from build123d import *

# Parameters (mm, degrees)
BOSS_EXTRUDE1_DEPTH = 0.75
BOSS_EXTRUDE2_DEPTH = 0.5
CUT_EXTRUDE1_DEPTH  = 0.1
CUT_EXTRUDE2_DEPTH  = 0.2
SKETCH5_W           = 0.45
SKETCH5_H           = 0.6
SKETCH6_W           = 0.45
SKETCH6_H           = 0.6
SKETCH7_W           = 1.25
SKETCH7_H           = 0.5
HOLE1_D             = 0.9
HOLE1_DEPTH         = 1.85
HOLE1_CBORE_D       = 2.5
HOLE1_CBORE_DEPTH   = 0.75
FILLET1_R           = 0.1
CHAMFER1_SIZE       = 0.15
FILLET2_R           = 0.25
FILLET3_R           = 1


with BuildPart() as part:
    # Sketch1 → Boss-Extrude1 (new body)
    with BuildSketch(Plane(origin=(0, 0, 0), x_dir=(-1, 0, 0), z_dir=(0, 0, -1))):
        with BuildLine():
            Line((-18.147160188, -0.321056231), (-16.640459832, -0.807555039))
            ThreePointArc((-16.640459832, -0.807555039), (-14.376672703, 1.830313994), (-11.123104682, 3.053988922))
            Line((-11.123104682, 3.053988922), (-11.854774008, 4.687962623))
            Line((-11.854774008, 4.687962623), (-11.980143643, 8.966094329))
            Line((-11.980143643, 8.966094329), (-13.651153285, 11.372867219))
            ThreePointArc((-13.651153285, 11.372867219), (-13.886856414, 11.501581597), (-14.131154362, 11.390038472))
            ThreePointArc((-14.131154362, 11.390038472), (-17.168571063, 5.887500969), (-18.147160188, -0.321056231))
        make_face()
    extrude(amount=-BOSS_EXTRUDE1_DEPTH)

    # Sketch2 → Boss-Extrude2 (add)
    with BuildSketch(Plane.XY.offset(0.75)):
        with BuildLine():
            Line((18.147160188, -0.321056231), (16.196912485, -0.950772139))
            Line((16.196912485, -0.950772139), (13.090029226, -4.428012343))
            Line((13.090029226, -4.428012343), (12.448174494, -4.428012343))
            ThreePointArc((12.448174494, -4.428012343), (9.659124877, -5.936170482), (8.400603878, -3.02593619))
            Line((8.400603878, -3.02593619), (11.854774008, 4.687962623))
            Line((11.854774008, 4.687962623), (11.980143643, 8.966094329))
            Line((11.980143643, 8.966094329), (13.651153285, 11.372867219))
            ThreePointArc((13.651153285, 11.372867219), (13.886856414, 11.501581597), (14.131154362, 11.390038472))
            ThreePointArc((14.131154362, 11.390038472), (17.168571063, 5.887500969), (18.147160188, -0.321056231))
        make_face()
    extrude(amount=BOSS_EXTRUDE2_DEPTH)

    # Sketch3 → Cut-Extrude1 (cut)
    with BuildSketch(Plane.XY.offset(1.25)):
        with BuildLine():
            Line((11.118831997, 2.571420588), (10.212805559, -1.893755119))
            Line((10.212805559, -1.893755119), (9.327068413, -3.204862093))
            ThreePointArc((9.327068413, -3.204862093), (11.06260071, -2.868815002), (11.3986478, -4.604347299))
            Line((11.3986478, -4.604347299), (12.284384946, -3.293240325))
            Line((12.284384946, -3.293240325), (16.088661421, -0.786019055))
            ThreePointArc((16.088661421, -0.786019055), (14.012715525, 1.498074346), (11.118831997, 2.571420588))
        make_face()
    extrude(amount=-CUT_EXTRUDE1_DEPTH, mode=Mode.SUBTRACT)

    # Sketch4 → Cut-Extrude2 (cut)
    with BuildSketch(Plane.XY.offset(1.15)):
        with BuildLine():
            Line((11.006450661, -0.718966828), (9.327068413, -3.204862093))
            ThreePointArc((9.327068413, -3.204862093), (11.06260071, -2.868815002), (11.3986478, -4.604347299))
            Line((11.3986478, -4.604347299), (13.078030048, -2.118452035))
            ThreePointArc((13.078030048, -2.118452035), (12.182188875, -1.211551493), (11.006450661, -0.718966828))
        make_face()
    extrude(amount=-CUT_EXTRUDE2_DEPTH, mode=Mode.SUBTRACT)

    # Sketch5 → Revolve1 (revolve)
    with BuildSketch(Plane(origin=(0, 0.611982068, 0), x_dir=(1, 0, 0), z_dir=(0, 1, 0))):
        with Locations((17.216029708, 0.3)):
            Rectangle(SKETCH5_W, SKETCH5_H)
    revolve(axis=Axis((16.991029708, 0.611982068, -0.6), (0, 0, 1)))

    # Sketch6 → Revolve2 (revolve)
    with BuildSketch(Plane(origin=(0, 8.246041644, 0), x_dir=(1, 0, 0), z_dir=(0, 1, 0))):
        with Locations((14.535071469, 0.3)):
            Rectangle(SKETCH6_W, SKETCH6_H)
    revolve(axis=Axis((14.310071469, 8.246041644, -0.6), (0, 0, 1)))

    # Sketch7 → Cut-Revolve1 (revolve, cut)
    with BuildSketch(Plane.XZ.offset(3.904604696)):
        with Locations((10.987858107, 1)):
            Rectangle(SKETCH7_W, SKETCH7_H)
    revolve(axis=Axis((10.362858107, -3.904604696, 1.25), (0, 0, -1)), mode=Mode.SUBTRACT)

    # Hole1
    with Locations(Plane.XY.offset(1.25)):
        with Locations((15.524716589, 3.231351436)):
            CounterBoreHole(HOLE1_D / 2, HOLE1_CBORE_D / 2, HOLE1_CBORE_DEPTH, depth=HOLE1_DEPTH)

    # Fillet1
    fillet1_edges = [part.edges().sort_by_distance(p)[0] for p in [
        (13.860071469, 8.246041644, -0.6),
        (11.854774008, 4.687962623, 0.625),
        (12.448174494, -4.428012343, 1),
        (16.541029708, 0.611982068, -0.6),
        (11.980143643, 8.966094329, 0.625),
        (13.090029226, -4.428012343, 1),
        (18.147160188, -0.321056231, 0.625),
        (16.196912485, -0.950772139, 1),
    ]]
    fillet(fillet1_edges, radius=FILLET1_R)

    # Chamfer1
    chamfer1_edges = [part.edges().sort_by_distance(p)[0] for p in [
        (14.274716589, 3.231351436, 1.25),
    ]]
    chamfer(chamfer1_edges, length=CHAMFER1_SIZE)

    # Fillet2
    fillet2_edges = [part.edges().sort_by_distance(p)[0] for p in [
        (13.078030048, -2.118452035, 1.05),
        (11.006450661, -0.718966828, 1.05),
    ]]
    fillet(fillet2_edges, radius=FILLET2_R)

    # Fillet3
    fillet3_edges = [part.edges().sort_by_distance(p)[0] for p in [
        (11.118831997, 2.571420588, 1.2),
        (16.088661421, -0.786019055, 1.2),
    ]]
    fillet(fillet3_edges, radius=FILLET3_R)


solid = part.part
The listing builds one solid part. Answer for the finished solid, in the listing's coordinates (mm). A direction names the side the tool comes from. Coordinates: 2 decimals unless noted, no trailing zeros. Loops run counter-clockwise (first coordinate to the right, second up) from the corner with the lowest first, then second, coordinate; pieces in that order, holes last.
1) Find section A-A on x = 17.75. Write down the section's boundary in (y, z).
2) Flat-ended cylindrical pins translate along their axes: pin 1 Ø1.8 at (x, y) = (11.5, -3.5) entering from +Z; pin 2 Ø3.5 at (x, y) = (15, 3.5) entering from -Z; pin 3 Ø2.5 at (x, y) = (12.5, 0) entering from -Z; pin 4 Ø1 at (x, z) = (11, 1) entering from +Y. Find the tip coordinate at first contact, or state that the pin passes through.
3) Find the intervals of material crossed by L1, parallel to Z at x = 14.75, y = 1; L2, parallel to Y at x = 15.25, z = 0.55; L3, parallel to X at y = -4.75, z = 0.9, in increasing order.
4) Find section B-B on y = 6.5. Write down the section's boundary in (x, z), then the cut area to 3 significant figures.
5) Determine the mould class of faces 1 (the face through (15.36, 4.47, 0.8)), 2 (the face through (15, 5, 0)), 3 (the face through (14.42, 1.8, 0.37)) for opening direction X: pulls with the +X half, pulls with the -X half, needs draft (parallel to the pull), parting line crosses it, or undercut.
6) A tool of negligible diameter and unlimited length cuts with its end or side. For faces 4 (the face through (12.813, 10.165, 0.616)), 5 (the face through (13, 0, 1.15)), 6 (the face through (12, -1, 0.75)), 7 (the face through (13.86, 8.27, -0.25)), 8 (the face through (13, 3, 1.25)), from which of +Z, -Z, +X, -X, +Y, -Y can it reach the whole face along a straight path? Write none if from no direction.
Values:
1. outline: (-0.45, 0) - (3.79, 0) - (3.79, 1.25) - (-0.45, 1.25) - close
2. pin 1: stops at z = 1.25
2. pin 2: stops at z = 0
2. pin 3: stops at z = 0.75
2. pin 4: stops at y = 3.9
3. L1: z = 0.75 to 1.25
3. L2: y = 1.11 to 2.01, 4.45 to 9.84
3. L3: x = 8.39 to 9.44, 11.28 to 12.34
4. outline: (11.91, 0) - (16.95, 0) - (16.95, 1.25) - (11.91, 1.25) - close
4. area: 6.30 mm2
5. face 1: undercut
5. face 2: needs draft
5. face 3: pulls with the -X half
6. face 4: +Z, -Z, -X, +Y
6. face 5: +Z
6. face 6: -Z, -X, -Y
6. face 7: -Z
6. face 8: +Z, +X, -X, +Y, -Y
